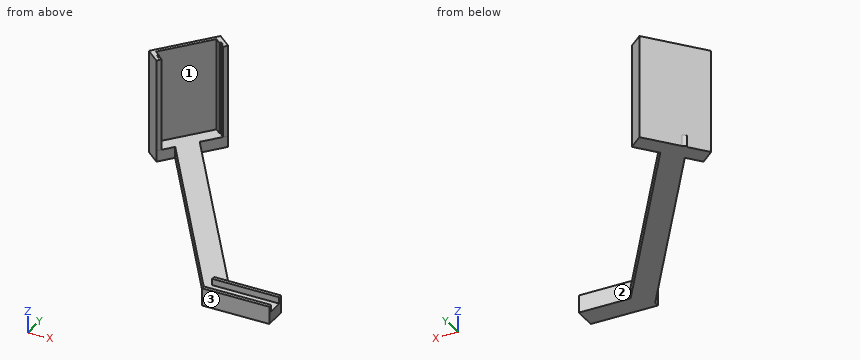
from build123d import *

# Parameters (mm, degrees)
CROQUIS_PLACA_CLIP_W = 30
CROQUIS_PLACA_CLIP_H = 9.9
PLACA_CLIP_DEPTH     = 5
CROQUIS_MORDAZAS_W   = 30
CROQUIS_MORDAZAS_H   = 1.6
MORDAZAS_DEPTH       = 2.9
BRAZO_DEPTH          = 5
TOPE_CUNA_DEPTH      = 5
CUNA_DEPTH           = 46.5


with BuildPart() as part:
    # Croquis_placa_clip → Placa_clip (new body)
    with BuildSketch(Plane.XY.offset(-133.1)):
        with Locations((-39, 79.75)):
            Rectangle(CROQUIS_PLACA_CLIP_W, CROQUIS_PLACA_CLIP_H)
    extrude(amount=PLACA_CLIP_DEPTH)

    # Croquis_mordazas → Mordazas (add)
    with BuildSketch(Plane.XY.offset(-128.1)):
        with Locations((-39, 83.9)):
            Rectangle(CROQUIS_MORDAZAS_W, CROQUIS_MORDAZAS_H)
        with Locations((-39, 75.6)):
            Rectangle(CROQUIS_MORDAZAS_W, CROQUIS_MORDAZAS_H)
    extrude(amount=MORDAZAS_DEPTH)

    # Croquis_brazo → Brazo (add)
    with BuildSketch(Plane.XY.offset(-133.1)):
        Polygon((-54.136621543, 77.191377169), (-121.944749796, 177.06116426), (-113.671506709, 182.678409922), (-45.863378457, 82.808622831), align=None)
    extrude(amount=BRAZO_DEPTH)

    # Croquis_tope → Tope_cuna (add)
    with BuildSketch(Plane.XY.offset(-133.1)):
        Polygon((-128.196522897, 168.676764411), (-108.647880385, 192.088312329), (-102.507146505, 186.960799539), (-122.055789016, 163.549251621), align=None)
    extrude(amount=TOPE_CUNA_DEPTH)

    # Croquis_cuna → Cuna (add)
    with BuildSketch(Plane.XY.offset(-133.1)):
        Polygon((-108.647880385, 192.088312329), (-102.507146505, 186.960799539), (-103.917212522, 185.272097722), (-105.145359298, 186.29760028), (-104.760795839, 186.758155321), (-106.142460962, 187.911845699), (-106.655212241, 187.297772311), (-108.957987446, 189.220589607), (-125.430122284, 169.493482017), (-123.127347079, 167.570664721), (-123.640098358, 166.956591333), (-122.258433235, 165.802900955), (-121.873869775, 166.263455996), (-120.645722999, 165.237953438), (-122.055789016, 163.549251621), (-128.196522897, 168.676764411), align=None)
    extrude(amount=CUNA_DEPTH)


solid = part.part
Can you work these out from the model? Positions are in its coordinate system, mm. Face numbers are marked on the shaded views. Round coordinates to 2 decimals unless told otherwise and drop trailing zeros. Order: outer loops, then holes, each group sorted by start corner. A loop starts at its lowest first (then second) coordinate and runs counter-clockwise, first axis right, second up. Notation, with made-up numbers: (-31, 54) -> (1, 54) arc R21 ccw to (1, 82) -> close; hole circle Ø1 at (29.5, 55). An arc over 180 degrees is marked (long way). Write each question's results on one line, items separated by ' | '. Start each with the question number.
Item 1: Please list where these lines run through material, in increasing order: L1, parallel to Z at x = -29.5, y = 82; L2, parallel to Y at x = -106.5, z = -130; L3, parallel to X at y = 181, z = -106.
Item 2: Will these pins go through, and if not, where does the flat tip stop? pin 1 (0.5 mm diameter, centred on x = -31.5, y = 83.5, fed in from +Z); pin 2 (0.5 mm diameter, centred on y = 83.5, z = -126.5, fed in from -X); pin 3 (10 mm diameter, centred on y = 167, z = -114.5, fed in from +X); pin 4 (6 mm diameter, centred on x = -95, y = 165, fed in from +Z).
Item 3: If we section it at D-D, the plane x = -112.5: Write out the boundary of the cut face in (y, z) (3 decimals), then the cut area to 3 significant figures.
Item 4: Thinking about a two-plate mould opening in Y: for the marked faces 1, 2 and 3, which applies, +Y half, -Y half, draft (parallel to the pull), parting line (faces both ways), or undercut?
Item 5: If we section it at C-C, the plane y = 183: Write out the boundary of the cut face in (x, z), then the cut area to 3 significant figures.
Item 6: If we section it at B-B, the plane x = -37.5: Write out the boundary of the cut face in (y, z).
Item 7: If we section it at A-A, the plane z = -110: Write out the boundary of the cut face in (x, y).
Results:
1) L1: z = -133.1 to -128.1 | L2: y = 154.31 to 172.12, 182.18 to 190.29 | L3: x = -117.91 to -115.82
2) pin 1: stops at z = -125.2 | pin 2: stops at x = -54 | pin 3: stops at x = -120.65 | pin 4: passes through
3) outline: (163.151, -133.1) -> (187.475, -133.1) -> (187.475, -86.6) -> (184.979, -86.6) -> (184.979, -128.1) -> (163.151, -128.1) -> close | area: 225 mm2
4) face 1: undercut | face 2: +Y half | face 3: -Y half
5) outline: (-116.24, -133.1) -> (-105.81, -133.1) -> (-105.81, -128.1) -> (-114.15, -128.1) -> (-114.15, -86.6) -> (-116.24, -86.6) -> close | area: 139 mm2
6) outline: (74.8, -133.1) -> (84.7, -133.1) -> (84.7, -125.2) -> (83.1, -125.2) -> (83.1, -128.1) -> (76.4, -128.1) -> (76.4, -125.2) -> (74.8, -125.2) -> close
7) outline: (-128.2, 168.68) -> (-122.06, 163.55) -> (-120.65, 165.24) -> (-121.87, 166.26) -> (-122.26, 165.8) -> (-123.64, 166.96) -> (-123.13, 167.57) -> (-125.43, 169.49) -> (-108.96, 189.22) -> (-106.66, 187.3) -> (-106.14, 187.91) -> (-104.76, 186.76) -> (-105.15, 186.3) -> (-103.92, 185.27) -> (-102.51, 186.96) -> (-108.65, 192.09) -> close
